Design review of the part built by this model. Coordinates are the model's own, in mm. Round coordinates to 2 decimals unless told otherwise and drop trailing zeros. Loops run counter-clockwise (first coordinate to the right, second up) from the corner with the lowest first, then second, coordinate; pieces in that order, holes last. Notation, with made-up numbers: (-23, 31) - (3, 31) arc R11 cw to (3, 49) - close; hole circle Ø8 at (75, -26). An arc over 180 degrees is marked (long way). Return JSON: item names as keys, results as strings. Group by question number.
(1) We need section A-A, the plane y = -0.5. Write out the cut boundary in (x, z), and give its area (3 significant figures).
(2) We need section C-C, the plane y = 13.25. Write out the cut boundary in (x, z).
(3) The part is to be moulded in two halves that separate along Z. For faces 1 (the cylindrical face through (-1.46, -0.74, -6.59)), 2 (the flat face through (3, -1.5, 0)), 3 (the cylindrical face through (0.067, 11.396, 0.183)), say which applies: pulls with the +Z half, pulls with the -Z half, needs draft (parallel to the pull), parting line crosses it, or undercut.
(4) We need section D-D, the plane z = -6. Write out the cut boundary in (x, y).
(5) We need section B-B, the plane z = 0.75. Give the number of separate pieces and of enclosed holes in the cut face, and give its area (3 significant figures).
(6) Clearance check with flat-ended pins moving along their axes: pin 1 (5 mm diameter, centred on x = 0, y = 4.5, fed in from -Z); pin 2 (1.5 mm diameter, centred on x = 5, y = 7, fed in from -Z); pin 3 (3 mm diameter, centred on y = 10, z = 0, fed in from +X). State where each tip first meets the part, or that it passes through.
(7) Wall thickness on L1, parallel to Y at x = 2.5, z = 6; L2, parallel to Z at x = 2, y = 0.25; L3, parallel to Z at x = 0, y = 7.25: over which ranges is each line inside the solid? List them lowest first. Write a range as [from, to].
from build123d import *

# Parameters (mm, degrees)
SKETCH3_R               = 6.75
BOSS_EXTRUDE1_DEPTH     = 1.5
SKETCH5_R               = 2.5
CUT_EXTRUDE1_DEPTH      = 11
SKETCH6_R               = 1.408145202
CUT_EXTRUDE2_DEPTH      = 7.75
CUT_EXTRUDE2_DEPTH_BACK = 7.75


with BuildPart() as part:
    # Sketch1 → Revolve1 (revolve)
    with BuildSketch(Plane.XY):
        with BuildLine():
            Line((0, 0), (-5.75, 0))
            add(Edge.make_bspline(
                [(-5.75, 0), (-5.385455056, 6.49991136), (-4.801363332, 8.498230235), (-4.241672522, 11.5)],
                knots=[0, 0, 0, 0, 1, 1, 1, 1], degree=3))
            ThreePointArc((-4.241672522, 11.5), (-2.749626601, 14.012035059), (0, 15))
            Line((0, 15), (0, 0))
        make_face()
    revolve(axis=Axis((0, 15, 0), (0, -1, 0)))

    # Sketch3 → Boss-Extrude1 (add)
    with BuildSketch(Plane.XZ):
        Circle(SKETCH3_R)
    extrude(amount=BOSS_EXTRUDE1_DEPTH)

    # Sketch5 → Cut-Extrude1 (cut)
    with BuildSketch(Plane.XZ.offset(1.5)):
        Circle(SKETCH5_R)
    extrude(amount=-CUT_EXTRUDE1_DEPTH, mode=Mode.SUBTRACT)

    # Sketch6 → Cut-Extrude2 (cut, two sides)
    with BuildSketch(Plane(origin=(0, 0, 0), x_dir=(0, 0, -1), z_dir=(1, 0, 0))) as cut_extrude2_sk:
        with Locations((0, 10)):
            Circle(SKETCH6_R)
    extrude(amount=CUT_EXTRUDE2_DEPTH, mode=Mode.SUBTRACT)
    extrude(cut_extrude2_sk.sketch, amount=-CUT_EXTRUDE2_DEPTH_BACK, mode=Mode.SUBTRACT)


solid = part.part
Solutions:
{
 "1": {"outline": "circle Ø13.5 at (0, 0); hole circle Ø5 at (0, 0)", "area": "124 mm^2"},
 "2": {"outline": "circle Ø6.95 at (0, 0)"},
 "3": {"face 1": "parting line crosses it", "face 2": "needs draft", "face 3": "undercut"},
 "4": {"outline": "(-3.09, -1.5) - (3.09, -1.5) - (3.09, 0) - (-3.09, 0) - close"},
 "5": {"separate pieces": "3", "enclosed holes": "0", "area": "88.5 mm^2"},
 "6": {"pin 1": "z = -5.62", "pin 2": "z = -2.8", "pin 3": "x = 4.82"},
 "7": {"L1": "[-1.5, 0]", "L2": "[-5.38, -1.5], [1.5, 5.38]", "L3": "[-5.04, -2.5], [2.5, 5.04]"}
}
